Work out the finished part from the listing and answer in its coordinate system (mm). Face numbers are marked on the shaded views. A direction names the side the tool comes from. Give positions to 0.01 mm unless a question says otherwise; leave off trailing zeros. Order: outer loops, then holes, each group sorted by start corner. A loop starts at its lowest first (then second) coordinate and runs counter-clockwise, first axis right, second up. Notation, with made-up numbers: (-23.75, -3) - (8.25, -3) arc R10 ccw to (8.25, 9) - close; hole circle Ø5 at (63.25, 31). An arc over 180 degrees is marked (long way). Write each question's results on one line, items separated by ' | '.
from build123d import *

# Parameters (mm, degrees)
SKETCH1_R           = 50
BOSS_EXTRUDE1_DEPTH = 7.5
SKETCH2_W           = 15
SKETCH2_H           = 15
BOSS_EXTRUDE2_DEPTH = 10
SKETCH3_R           = 1.75
CUT_EXTRUDE1_DEPTH  = 15
SKETCH4_R           = 3.3
CUT_EXTRUDE2_DEPTH  = 2.5
CUT_EXTRUDE3_DEPTH  = 2.5
SKETCH6_W           = 6.8
SKETCH6_H           = 6.8
CUT_EXTRUDE4_DEPTH  = 17.5


with BuildPart() as part:
    # Sketch1 → Boss-Extrude1 (new body)
    with BuildSketch(Plane(origin=(0, 0, 0), x_dir=(1, 0, 0), z_dir=(0, 1, 0))):
        with Locations(Location((0, 0, 0), (0, 0, 270))):
            Circle(SKETCH1_R)
    extrude(amount=BOSS_EXTRUDE1_DEPTH)

    # Sketch2 → Boss-Extrude2 (add)
    with BuildSketch(Plane(origin=(0, 7.5, 0), x_dir=(1, 0, 0), z_dir=(0, 1, 0))):
        Rectangle(SKETCH2_W, SKETCH2_H)
    extrude(amount=BOSS_EXTRUDE2_DEPTH)

    # Sketch3 → Cut-Extrude1 (cut)
    with BuildSketch(Plane(origin=(7.5, 0, 0), x_dir=(0, 0, -1), z_dir=(1, 0, 0))):
        with Locations((0, 12.5)):
            Circle(SKETCH3_R)
    extrude(amount=-CUT_EXTRUDE1_DEPTH, mode=Mode.SUBTRACT)

    # Sketch4 → Cut-Extrude2 (cut)
    with BuildSketch(Plane(origin=(7.5, 0, 0), x_dir=(0, 0, -1), z_dir=(1, 0, 0))):
        with Locations((0, 12.5)):
            Circle(SKETCH4_R)
    extrude(amount=-CUT_EXTRUDE2_DEPTH, mode=Mode.SUBTRACT)

    # Sketch5 → Cut-Extrude3 (cut)
    with BuildSketch(Plane.ZY.offset(7.5)):
        Polygon((-3.35, 12.5), (-1.675, 9.598814897), (1.675, 9.598814897), (3.35, 12.5), (1.675, 15.401185103), (-1.675, 15.401185103), align=None)
    extrude(amount=-CUT_EXTRUDE3_DEPTH, mode=Mode.SUBTRACT)

    # Sketch6 → Cut-Extrude4 (cut)
    with BuildSketch(Plane(origin=(0, 17.5, 0), x_dir=(1, 0, 0), z_dir=(0, 1, 0))):
        Rectangle(SKETCH6_W, SKETCH6_H)
    extrude(amount=-CUT_EXTRUDE4_DEPTH, mode=Mode.SUBTRACT)


solid = part.part
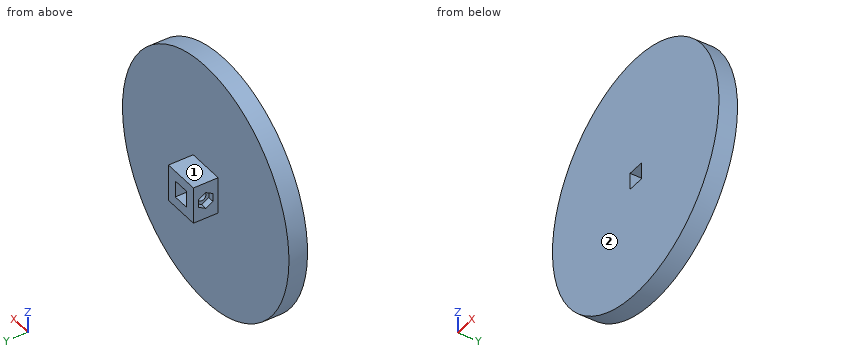
1. Straight lines are drawn through the part: line 1 (Y direction, x = 4, z = 0); line 2 (Y direction, x = 6.4, z = 0); line 3 (X direction, y = 14.5, z = 3). For each, find the intervals that lie inside material, in ascending order. Write a range as [from, to].
Answer list:
line 1: [0, 10.75], [14.25, 17.5] | line 2: [0, 9.2], [15.8, 17.5] | line 3: [-7.5, -3.4], [3.4, 7.5]
2. A cutting plane is placed at C-C, the plane y = 3.75. Write down the section's boundary in (x, z), then the cut area to 3 significant figures.
Answer list:
outline: circle Ø100 at (0, 0); hole (-3.4, -3.4) - (3.4, -3.4) - (3.4, 3.4) - (-3.4, 3.4) - close | area: 7,810 mm^2
3. A cutting plane is placed at D-D, the plane z = 31. Write down the section's boundary in (x, y), then the cut area to 3 significant figures.
Answer list:
outline: (-39.23, 0) - (39.23, 0) - (39.23, 7.5) - (-39.23, 7.5) - close | area: 588 mm^2
4. Given P1, Ø10, axis at x = -39.5, y = 8, coming from the -Z side; P2, Ø10, axis at x = 9.5, y = 15, coming from the -Z side; P3, Ø3, axis at x = 34.5, z = 26.5, coming from the +Y side, each flat-ended and moving along its own axis, determine where each tip first touches the part or whether it passes through.
Answer list:
P1: z = -36.17 | P2: z = -7.5 | P3: y = 7.5
5. A cutting plane is placed at B-B, the plane x = 0. Write down the section's boundary in (y, z).
Answer list:
outline: (0, -50) - (7.5, -50) - (7.5, -7.5) - (17.5, -7.5) - (17.5, -3.4) - (0, -3.4) - close; (0, 3.4) - (17.5, 3.4) - (17.5, 7.5) - (7.5, 7.5) - (7.5, 50) - (0, 50) - close
6. A tool of negligible diameter and unlimited length cuts with its end or side. For the marked faces 1 and 2, from which of +Z, -Z, +X, -X, +Y, -Y can it reach the whole face along a straight path? Write none if from no direction.
Answer list:
face 1: +Z, +X, -X, +Y | face 2: +Z, -Z, +X, -X, -Y
7. A cutting plane is placed at A-A, the plane z = 0. Write down the section's boundary in (x, y).
Answer list:
outline: (-50, 0) - (-3.4, 0) - (-3.4, 10.75) - (-5, 10.75) - (-5, 9.6) - (-7.5, 9.6) - (-7.5, 7.5) - (-50, 7.5) - close; (-7.5, 15.4) - (-5, 15.4) - (-5, 14.25) - (-3.4, 14.25) - (-3.4, 17.5) - (-7.5, 17.5) - close; (3.4, 0) - (50, 0) - (50, 7.5) - (7.5, 7.5) - (7.5, 9.2) - (5, 9.2) - (5, 10.75) - (3.4, 10.75) - close; (3.4, 14.25) - (5, 14.25) - (5, 15.8) - (7.5, 15.8) - (7.5, 17.5) - (3.4, 17.5) - close
